from build123d import *

# Parameters (mm, degrees)
F0_R     = 63.5
F0_R_2   = 5.08
F1_DEPTH = 31.75
F2_R     = 44.9082532623
F3_DEPTH = 5.08
F4_R     = 17.386039325
F5_DEPTH = 5.08
F7_D     = 10.3
F7_DEPTH = 81.4578
F7_TIP   = 3.094432188


with BuildPart() as f1:
    # F0 (on Front) → F1 (new body)
    with BuildSketch(Plane.XZ):
        Circle(F0_R)
        with Locations((-47.3893386877, -27.3602474481)):
            Circle(F0_R_2, mode=Mode.SUBTRACT)
        with Locations((0, -54.7204948962)):
            Circle(F0_R_2, mode=Mode.SUBTRACT)
        with Locations((47.3893386877, -27.3602474481)):
            Circle(F0_R_2, mode=Mode.SUBTRACT)
        with Locations((-47.3893386877, 27.3602474481)):
            Circle(F0_R_2, mode=Mode.SUBTRACT)
        with Locations((47.3893386877, 27.3602474481)):
            Circle(F0_R_2, mode=Mode.SUBTRACT)
        with Locations((0, 54.7204948962)):
            Circle(F0_R_2, mode=Mode.SUBTRACT)
    extrude(amount=F1_DEPTH)

    # F2 (on face) → F3 (cut)
    with BuildSketch(Plane.XZ.offset(31.75)):
        Circle(F2_R)
    extrude(amount=-F3_DEPTH, mode=Mode.SUBTRACT)

    # F4 (on face) → F5 (join)
    with BuildSketch(Plane.XZ.offset(26.67)):
        Circle(F4_R)
    extrude(amount=F5_DEPTH)

    # F7
    with Locations(Plane.XZ.offset(31.75)):
        with Locations((0, 0)):
            Hole(F7_D / 2, depth=F7_DEPTH)
            with Locations((0, 0, -(F7_DEPTH + F7_TIP / 2))):  # 118° drill point
                Cone(0, F7_D / 2, F7_TIP, mode=Mode.SUBTRACT)


solid = f1.part
Verification items for the finished model (mm, model axes). A direction names the side the tool comes from. Round coordinates to 2 decimals unless told otherwise and drop trailing zeros. Loops run counter-clockwise (first coordinate to the right, second up) from the corner with the lowest first, then second, coordinate; pieces in that order, holes last. Notation, with made-up numbers: (14.5, 49.25) - (54.5, 49.25) arc R14 ccw to (54.5, 59.25) - close; hole circle Ø5 at (43, 66). An arc over 180 degrees is marked (long way). Use a Markdown table: item, result. Add a question column.
1. Section check B-B, the plane z = 0. Record the boundary of the cut face in (x, y), plus the area to 3 significant figures.
2. Section check C-C, the plane x = 48. Record the boundary of the cut face in (y, z).
3. Section check A-A, the plane x = 0. Record the boundary of the cut face in (y, z).
4. Thickness scan on probe 1 along Z at (x, y) = (0, -30.15); probe 2 along Z at (x, y) = (2.5, -8); probe 3 along Y at (x, z) = (-30, -30). Record the ranges inside material, lowest first. Write a range as [from, to].
5. Section check D-D, the plane z = 38.5. Record the boundary of the cut face in (x, y), plus the area to 3 significant figures.
6. Gauge pin test, flat ends, axial feed: pin 1 (8 mm diameter, centred on x = 35.5, y = -24.5, fed in from +Z); pin 2 (5 mm diameter, centred on y = -4, z = -33.5, fed in from -X); pin 3 (1 mm diameter, centred on x = 31.5, y = -28, fed in from -Z); pin 4 (8 mm diameter, centred on x = 0, z = 0, fed in from -Y). Record the tip position at first contact, or that the pin passes through.
7. Access from +Z, -Z, +X, -X, +Y, -Y to the whole of each face (thin tool, end or side, straight path). Record for faces 1 (the face through (-35.638, -29.246, -27.326)), 2 (the face through (2.34, -15.65, 50.21)).
8. Release check for a two-part mould opening along X. For faces 3 (the face through (42.314, -15.653, -27.137)), 4 (the face through (-13.77, -15.65, -61.99)), 5 (the face through (4, -31.75, 4)) record: released by +X, released by -X, zero draft, split by the parting line, or undercut.
Checks:
| question | item | result |
|---|---|---|
| 1 | outline | (-63.5, -31.75) - (-44.91, -31.75) - (-44.91, -26.67) - (-17.39, -26.67) - (-17.39, -31.75) - (-5.15, -31.75) - (-5.15, 0) - (-63.5, 0) - close; (5.15, -31.75) - (17.39, -31.75) - (17.39, -26.67) - (44.91, -26.67) - (44.91, -31.75) - (63.5, -31.75) - (63.5, 0) - (5.15, 0) - close |
| 1 | area | 3,430 mm^2 |
| 2 | outline | (-31.75, -41.57) - (0, -41.57) - (0, -32.4) - (-31.75, -32.4) - close; (-31.75, -22.32) - (0, -22.32) - (0, 22.32) - (-31.75, 22.32) - close; (-31.75, 32.4) - (0, 32.4) - (0, 41.57) - (-31.75, 41.57) - close |
| 3 | outline | (-31.75, -63.5) - (0, -63.5) - (0, -59.8) - (-31.75, -59.8) - close; (-31.75, -49.64) - (0, -49.64) - (0, -5.15) - (-31.75, -5.15) - (-31.75, -17.39) - (-26.67, -17.39) - (-26.67, -44.91) - (-31.75, -44.91) - close; (-31.75, 5.15) - (0, 5.15) - (0, 49.64) - (-31.75, 49.64) - (-31.75, 44.91) - (-26.67, 44.91) - (-26.67, 17.39) - (-31.75, 17.39) - close; (-31.75, 59.8) - (0, 59.8) - (0, 63.5) - (-31.75, 63.5) - close |
| 4 | probe 1 | z = [-63.5, -59.8], [-49.64, -44.91], [-17.39, -5.15], [5.15, 17.39], [44.91, 49.64], [59.8, 63.5] |
| 4 | probe 2 | z = [-63.45, -59.14], [-50.3, -4.5], [4.5, 50.3], [59.14, 63.45] |
| 4 | probe 3 | y = [-26.67, 0] |
| 5 | outline | (-50.5, -31.75) - (-23.12, -31.75) - (-23.12, -26.67) - (23.12, -26.67) - (23.12, -31.75) - (50.5, -31.75) - (50.5, 0) - (-50.5, 0) - close |
| 5 | area | 2,970 mm^2 |
| 6 | pin 1 | stops at z = 55.14 |
| 6 | pin 2 | stops at x = -55.42 |
| 6 | pin 3 | stops at z = -55.42 |
| 6 | pin 4 | passes through |
| 7 | face 1 | -Y |
| 7 | face 2 | +Y, -Y |
| 8 | face 3 | undercut |
| 8 | face 4 | split by the parting line |
| 8 | face 5 | zero draft |
